For this review, use the dimensioned drawing (mm, ordinates from the lowest corner) and the shaded views. A direction names the side the tool comes from. Round coordinates to 2 decimals unless told otherwise and drop trailing zeros. Order: outer loops, then holes, each group sorted by start corner. A loop starts at its lowest first (then second) coordinate and runs counter-clockwise, first axis right, second up. Notation, with made-up numbers: M -30,-1 L 11,-1 A29 ccw 11,37 Z; hole C 75,88 d4. An arc over 180 degrees is marked long. One line per item, written item: value. Start each with the question number.
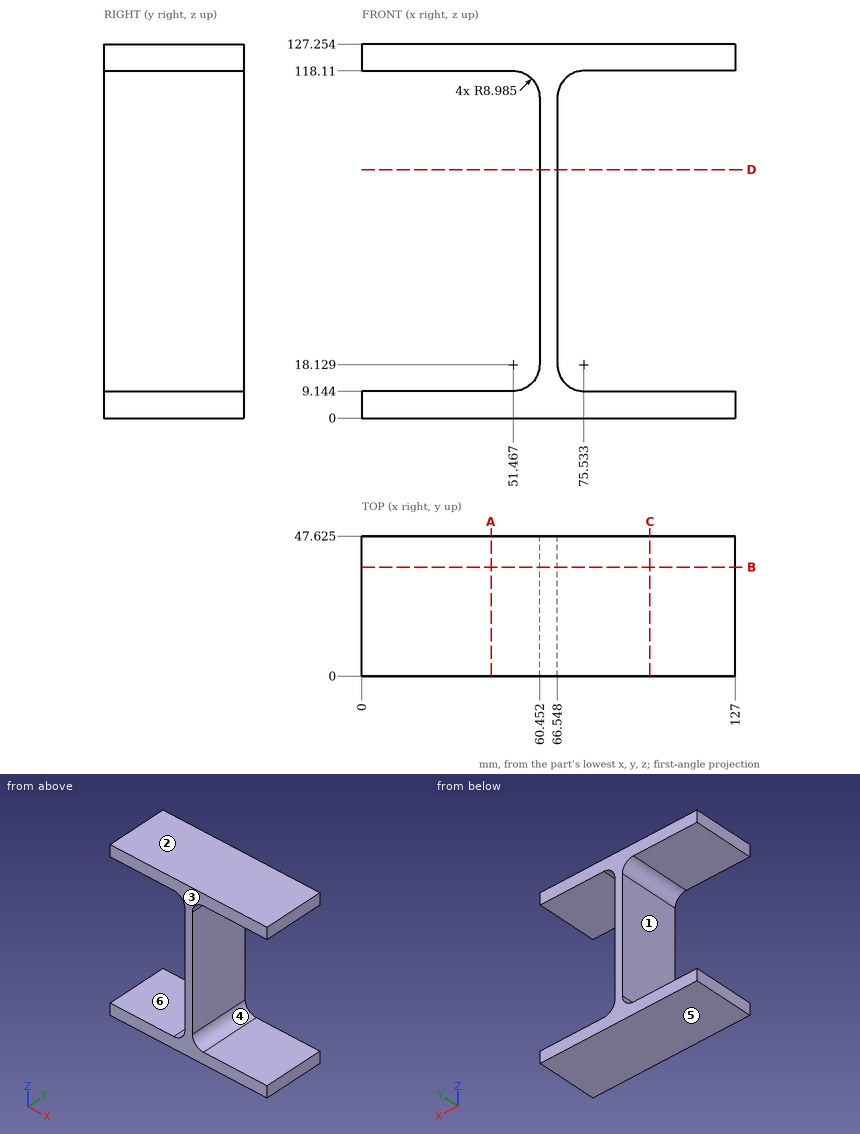
Item 1: Consider section A-A, the plane x = 44. Give the boundary of the cut face in (y, z) (1 decimal), then the cut area to 3 significant figures.
Item 2: Wall thickness on L1, parallel to Z at x = 40.5, y = 8.5; L2, parallel to X at y = 31.5, z = 103; L3, parallel to Z at x = 55, y = 28.5 (1 decimal): over which ranges is each line inside the solid? List them lowest first.
Item 3: Clearance check with flat-ended pins moving along their axes: P1, Ø10, axis at y = 38.5, z = 85, coming from the +X side; P2, Ø24, axis at y = 28.5, z = 77.5, coming from the -X side; P3, Ø1.5, axis at y = 25, z = 15.5, coming from the +X side. State where each tip first meets the part, or that it passes through.
Item 4: The part is to be moulded in two halves that separate along Z. For the marked faces 1, 2 and 3, say which applies: pulls with the +Z half, pulls with the -Z half, needs draft (parallel to the pull), parting line crosses it, or undercut.
Item 5: Consider section B-B, the plane y = 37. Give the boundary of the cut face in (x, z) (1 decimal).
Item 6: Consider section D-D, the plane z = 84.5. Give the boundary of the cut face in (x, y) (1 decimal).
Item 7: Machinability: for the marked faces 4, 5 and 6, which of the approach directions +Z, -Z, +X, -X, +Y, -Y give a long, thin tool a straight path to every point of the face, cutting with its end or side? Answer none if there is none.
Computed:
1. outline: M 0,0 L 47.6,0 L 47.6,9.1 L 0,9.1 Z; M 0,118.1 L 47.6,118.1 L 47.6,127.3 L 0,127.3 Z
1. area: 871 mm^2
2. L1: z = 0 to 9.14, 118.11 to 127.25
2. L2: x = 60.45 to 66.55
2. L3: z = 0 to 9.9, 117.4 to 127.3
3. P1: stops at x = 66.55
3. P2: stops at x = 60.45
3. P3: stops at x = 67.21
4. face 1: undercut
4. face 2: pulls with the +Z half
4. face 3: needs draft
5. outline: M 0,0 L 127,0 L 127,9.1 L 75.5,9.1 A9 cw 66.5,18.1 L 66.5,109.1 A9 cw 75.5,118.1 L 127,118.1 L 127,127.3 L 0,127.3 L 0,118.1 L 51.5,118.1 A9 cw 60.5,109.1 L 60.5,18.1 A9 cw 51.5,9.1 L 0,9.1 Z
6. outline: M 60.5,0 L 66.5,0 L 66.5,47.6 L 60.5,47.6 Z
7. face 4: +X, +Y, -Y
7. face 5: -Z, +X, -X, +Y, -Y
7. face 6: -X, +Y, -Y
